```python
from build123d import *

# Parameters (mm, degrees)
F0_W     = 85
F0_H     = 40
F0_R     = 10
F1_DEPTH = 40
F2_R     = 12.5
F3_DEPTH = 40.001
F4_R     = 3
F5_DEPTH = 25
F6_R     = 3
F7_DEPTH = 25


with BuildPart() as f1:
    # F0 (on Front) → F1 (new body)
    with BuildSketch(Plane.XZ):
        with Locations((42.5, 20)):
            Rectangle(F0_W, F0_H)
        with Locations((60, 20)):
            Circle(F0_R, mode=Mode.SUBTRACT)
    extrude(amount=F1_DEPTH)

    # F2 (on face) → F3 (cut, through all)
    with BuildSketch(Plane.XY.offset(40)):
        with Locations((32.5, -20)):
            Circle(F2_R)
    extrude(amount=-F3_DEPTH, mode=Mode.SUBTRACT)

    # F4 (on face) → F5 (cut)
    with BuildSketch(Plane.YZ.offset(85)):
        with Locations((-20, 20)):
            Circle(F4_R)
    extrude(amount=-F5_DEPTH, mode=Mode.SUBTRACT)

    # F6 (on face) → F7 (cut)
    with BuildSketch(Plane(origin=(0, 0, 0), x_dir=(0, -1, 0), z_dir=(-1, 0, 0))):
        with Locations((20, 20)):
            Circle(F6_R)
    extrude(amount=-F7_DEPTH, mode=Mode.SUBTRACT)


solid = f1.part
```
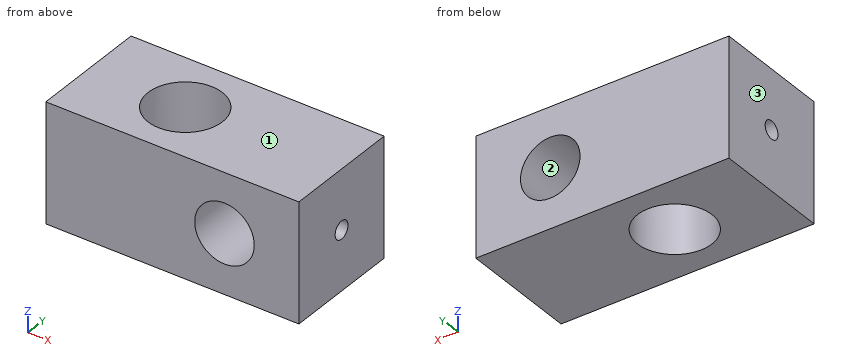
Geometry: final body of the model. Coordinates: model frame, mm. Face numbers are marked on the shaded views. Give positions to 0.01 mm unless a question says otherwise; leave off trailing zeros. Write each loop counter-clockwise with the first axis right and the second up, starting at its lowest first coordinate (ties: lowest second). Pieces come first, ordered by that corner, then holes.
1. Line query: probe 1 along Z at (x, y) = (77.25, -20); probe 2 along Y at (x, z) = (32, 28); probe 3 along Y at (x, z) = (8, 20). Output: solid intervals per line, ascending.
2. Section query D-D, the plane z = 15. Return loops of the section in (x, y).
3. Section query C-C, the plane x = 60. Return loops of the section in (y, z), then the cut area to 3 significant figures.
4. Pin query (flat end, axial travel): P1, Ø5, axis at y = -20, z = 20, coming from the +X side; P2, Ø5, axis at y = -20, z = 20, coming from the -X side. Return the tip coordinate at first contact, or that it passes through.
5. Section query A-A, the plane z = 20. Return loops of the section in (x, y), then the cut area to 3 significant figures.
6. Section query B-B, the plane y = -20. Return loops of the section in (x, z), then the cut area to 3 significant figures.
7. Draft query along X for the marked faces 1, 2 and 3. Return one class per face: released by +X, released by -X, zero draft, split by the parting line, or undercut.
Computed:
1. probe 1: z = 0 to 17, 23 to 40
1. probe 2: y = -40 to -32.49, -7.51 to 0
1. probe 3: y = -40 to -23, -17 to 0
2. outline: (0, -40) - (51.34, -40) - (51.34, 0) - (0, 0) - close; (68.66, -40) - (85, -40) - (85, 0) - (68.66, 0) - close; hole circle Ø25 at (32.5, -20)
3. outline: (-40, 0) - (0, 0) - (0, 10) - (-40, 10) - close; (-40, 30) - (0, 30) - (0, 40) - (-40, 40) - close
3. area: 800 mm2
4. P1: stops at x = 50.32
4. P2: stops at x = 44.75
5. outline: (0, -40) - (50, -40) - (50, 0) - (0, 0) - (0, -17) - (20.37, -17) arc R12.5 cw (long way) to (20.37, -23) - (0, -23) - close; (70, -40) - (85, -40) - (85, -23) - (70, -23) - close; (70, -17) - (85, -17) - (85, 0) - (70, 0) - close
5. area: 1,900 mm2
6. outline: (0, 0) - (20, 0) - (20, 17) - (0, 17) - close; (0, 23) - (20, 23) - (20, 40) - (0, 40) - close; (45, 0) - (85, 0) - (85, 17) - (69.54, 17) arc R10 cw (long way) to (69.54, 23) - (85, 23) - (85, 40) - (45, 40) - close
6. area: 1,870 mm2
7. face 1: zero draft
7. face 2: undercut
7. face 3: released by -X
